Can you work these out from the model? Positions are in its coordinate system, mm. Round coordinates to 2 decimals unless told otherwise and drop trailing zeros. Loops run counter-clockwise (first coordinate to the right, second up) from the corner with the lowest first, then second, coordinate; pieces in that order, holes last. Notation, with made-up numbers: (22.5, 27.5) - (44.5, 27.5) arc R28 ccw to (44.5, 54.5) - close; hole circle Ø6 at (87.5, -23.5). An arc over 180 degrees is marked (long way). Answer as CSV lines item,"result".
Autodesk Inventor part; units mm, degrees
ref_plane "YZ Plane" through (0, 0, 0) normal (1, 0, 0) x (0, 1, 0)
ref_plane "XY Plane" through (0, 0, 0) normal (0, 0, 1) x (1, 0, 0)
sketch "Sketch3" plane through (0, 0, 0) normal (1, 0, 0) x (0, 1, 0)
  line L0 (0, 0) -> (0, -30)
  line L1 (0, -30) -> (90, -30)
  line L2 (90, -30) -> (90, 0)
  line L3 (90, 0) -> (0, 0)
  line L4 (75, 0) -> (75, -14.9)
  line L5 (75, -14.9) -> (75.2, -14.9)
  line L6 (75.2, -14.9) -> (75.2, -15.1)
  line L7 (75.2, -15.1) -> (75, -15.1)
  line L8 (75, -15.1) -> (75, -30)
  dimension "d15" = 0.2
  dimension "d16" = 0.2
  dimension "d17" = 180
  dimension "d18" = 150
  dimension "d19" = 14.9
  dimension "d20" = 30
revolve "Revolution2" add sketch "Sketch3" angle 360 about axis through (0, 0, 0) along (0, 0, -1) contours L3 L2 L1 L8 L7 L6 L5 L4
ref_plane "Work Plane2" through (0, 90, 0) normal (0, 1, 0) x (-1, 0, 0)
sketch "Sketch4" plane through (0, 90, 0) normal (0, 1, 0) x (-1, 0, 0)
  line L0 (-75, -14.9) -> (75, -14.9)
  point P0 (0, 0)
  point P1 (0.0442, -15)
  dimension "d24" = 15
hole "Hole2" at (-0.0442, 90, -15) direction (0, -1, 0) diameter 2 depth 30 tip angle 118
properties part number "SFD_CuscinettoRadiale180x150x0.20" material "Stainless Steel"
Q1. Imagine slicing it at B-B (x = -42). Write out the boundary of the cut face in (y, z).
Checks:
outline,"(-79.6, -30) - (-62.14, -30) - (-62.14, -15.1) - (-62.38, -15.1) - (-62.38, -14.9) - (-62.14, -14.9) - (-62.14, 0) - (-79.6, 0) - close; (62.14, -30) - (79.6, -30) - (79.6, 0) - (62.14, 0) - (62.14, -14.9) - (62.38, -14.9) - (62.38, -15.1) - (62.14, -15.1) - close"
Q2. I'm going to push flat-ended pins straight in: pin 1 Ø1.5 at (y, z) = (56, -12) entering from -X; pin 2 Ø8 at (y, z) = (13.5, -12) entering from -X; pin 3 Ø12 at (x, y) = (63, 11) entering from +Z (3 decimals); pin 4 Ø8 at (x, z) = (15.5, -25.5) entering from -Y. Where does each tip first touch, or does it pass through?
Checks:
pin 1,"x = -71.05"
pin 2,"x = -89.5"
pin 3,"through"
pin 4,"y = -89.26"
Q3. Imagine slicing it at A-A (y = 0). Write out the boundary of the cut face in (x, z).
Checks:
outline,"(-90, -30) - (-75, -30) - (-75, -15.1) - (-75.2, -15.1) - (-75.2, -14.9) - (-75, -14.9) - (-75, 0) - (-90, 0) - close; (75, -30) - (90, -30) - (90, 0) - (75, 0) - (75, -14.9) - (75.2, -14.9) - (75.2, -15.1) - (75, -15.1) - close"
Q4. Imagine slicing it at C-C (z = -26). Write out the boundary of the cut face in (x, y).
Checks:
outline,"circle Ø180 at (0, 0); hole circle Ø150 at (0, 0)"
Q5. If I drill on line 1 along Z through (x, y) = (-70, -27); line 2 along X through (y, z) = (-1.5, -5) (1 decimal); line 3 along X through (y, z) = (0, -14.95), over which ranges is the centre line in solid material (lowest first)? Write a range as [from, to].
Checks:
line 1,"[-30, -15.1], [-14.9, 0]"
line 2,"[-90, -75], [75, 90]"
line 3,"[-90, -75.2], [75.2, 90]"
Q6. We'd pull the mould along X, two halves only. Please class faces 1 (the flat face through (74, -20, -30)), 2 (the cylindrical face through (74.362, -9.764, -22.654)), 3 (the cylindrical face through (79.845, 41.53, -14.79)): pulls with the +X half, pulls with the -X half, needs draft (parallel to the pull), parting line crosses it, or undercut.
Checks:
face 1,"needs draft"
face 2,"undercut"
face 3,"parting line crosses it"
